Verification items for the finished model (mm, model axes). A direction names the side the tool comes from. Give positions to 0.01 mm unless a question says otherwise; leave off trailing zeros. Loops run counter-clockwise (first coordinate to the right, second up) from the corner with the lowest first, then second, coordinate; pieces in that order, holes last. Notation, with made-up numbers: (62.5, 20.5) - (79.5, 20.5) arc R16 ccw to (79.5, 45.5) - close; hole circle Ø3 at (-27.5, 72). An arc over 180 degrees is marked (long way). Use one line per item in the form item = value.
```python
from build123d import *

# Parameters (mm, degrees)
SKETCH1_R                = 300
BOSS_EXTRUDE1_DEPTH      = 161
SKETCH2_R                = 192.75
SKETCH2_R_2              = 100
SKETCH2_W                = 642.75
SKETCH2_H                = 214
BOSS_EXTRUDE2_DEPTH      = 50
SKETCH3_R                = 75
CUT_EXTRUDE1_DEPTH       = 40
SKETCH4_R                = 100
CUT_EXTRUDE2_DEPTH       = 40
BOSS_EXTRUDE3_REACH      = 982.366
BOSS_EXTRUDE3_END_RADIUS = 192.75
SKETCH5_W                = 100
SKETCH5_H                = 83.75


with BuildPart() as part:
    # Sketch1 → Boss-Extrude1 (new body)
    with BuildSketch(Plane(origin=(0, 0, 0), x_dir=(1, 0, 0), z_dir=(0, 1, 0))):
        with Locations(Location((0, 0, 0), (0, 0, 270))):
            Circle(SKETCH1_R)
    extrude(amount=BOSS_EXTRUDE1_DEPTH)

    # Sketch2 → Boss-Extrude2 (add, symmetric)
    # profile 1 of 2: a face of its own
    with BuildSketch(Plane.XY):
        with Locations((330, 484)):
            Circle(SKETCH2_R)
        with Locations((330, 484)):
            Circle(SKETCH2_R_2, mode=Mode.SUBTRACT)
    # profile 2 of 2: a face of its own
    with BuildSketch(Plane.XY):
        with Locations((-201.375, 268)):
            Rectangle(SKETCH2_W, SKETCH2_H)
    extrude(amount=BOSS_EXTRUDE2_DEPTH, both=True)


with BuildPart() as boss_extrude2_piece_1:
    # of the separate pieces the step leaves, piece 1, a body of its own (boss_extrude2_pieces)
    add(part.part.solids().sort_by_distance((0, 0, 300))[0])

    # Sketch3 → Cut-Extrude1 (cut)
    with BuildSketch(Plane.XZ):
        with Locations(Location((0, 0, 0), (0, 0, 270))):
            Circle(SKETCH3_R)
    extrude(amount=-CUT_EXTRUDE1_DEPTH, mode=Mode.SUBTRACT)

    # Sketch4 → Cut-Extrude2 (cut)
    with BuildSketch(Plane.XZ.offset(-40)):
        with Locations(Location((0, 0, 0), (0, 0, 270))):
            Circle(SKETCH4_R)
    extrude(amount=-CUT_EXTRUDE2_DEPTH, mode=Mode.SUBTRACT)



with BuildPart() as boss_extrude2_piece_2:
    # of the separate pieces the step leaves, piece 2, a body of its own (boss_extrude2_pieces)
    add(part.part.solids().sort_by_distance((522.75, 484, -50))[0])


with BuildPart() as boss_extrude2_piece_1_1:
    add(boss_extrude2_piece_1.part)

    add(boss_extrude2_piece_2.part)  # Boss-Extrude3 merges Boss-Extrude2 piece 2
    # Boss-Extrude3: up to this cylinder (the profile starts outside it)
    boss_extrude3_end = Plane(origin=(330, 484, 0), z_dir=(0, 0, -1)) * Cylinder(BOSS_EXTRUDE3_END_RADIUS, 2351.232, mode=Mode.PRIVATE)
    # Sketch5 → Boss-Extrude3 (add, up to the surface)
    with BuildSketch(Plane(origin=(120, 0, 0), x_dir=(0, 0, -1), z_dir=(1, 0, 0)), mode=Mode.PRIVATE) as boss_extrude3_sk1:
        with Locations((0, 333.125)):
            Rectangle(SKETCH5_W, SKETCH5_H)
    boss_extrude3_tool1 = extrude(boss_extrude3_sk1.sketch, amount=BOSS_EXTRUDE3_REACH, mode=Mode.PRIVATE) - boss_extrude3_end
    add(boss_extrude3_tool1.solids().sort_by_distance((120, 333.125, 0))[0])


solid = boss_extrude2_piece_1_1.part
```
1. Section check A-A, the plane y = 484. Record the cut outline in (x, z).
Result set:
outline = (137.25, -50) - (230, -50) - (230, 50) - (137.25, 50) - close; (430, -50) - (522.75, -50) - (522.75, 50) - (430, 50) - close
2. Depth check by flat-ended pin: pin 1 Ø3 at (y, z) = (407.5, -7.5) entering from -X; pin 2 Ø4 at (x, z) = (-262, 78) entering from -Y; pin 3 Ø2 at (x, z) = (-403.5, 50.5) entering from -Y. Enter the tip coordinate at first touch or a pass-through.
Result set:
pin_1 = 152.44
pin_2 = 0
pin_3 = 161
3. Tool access check on faces 4 (the flat face through (-522.75, 267, 1)), 5 (the flat face through (-7, 358, -50)), 6 (the flat face through (1, 80, 1)), 7 (the flat face through (120, 225, 1)), 8 (the flat face through (-7, 358, 50)). Record the directions out of +Z, -Z, +X, -X, +Y, -Y that give a thin tool (end or side, any length) a straight path to the whole face; none if there is none.
Result set:
face_4 = +Z, -Z, -X, +Y, -Y
face_5 = -Z, +X, -X, +Y
face_6 = none
face_7 = +Z, -Z, +X
face_8 = +Z, +X, -X, +Y
4. Section check B-B, the plane z = 0. Record the cut outline in (x, y).
Result set:
outline = (-522.75, 161) - (-300, 161) - (-300, 0) - (-75, 0) - (-75, 40) - (-100, 40) - (-100, 80) - (100, 80) - (100, 40) - (75, 40) - (75, 0) - (300, 0) - (300, 161) - (120, 161) - (120, 291.25) - (330, 291.25) arc R192.75 ccw (long way) to (171.03, 375) - (-522.75, 375) - close; hole circle Ø200 at (330, 484)
5. Scan lines: probe 1 along X at (y, z) = (20, 0); probe 2 along Y at (x, z) = (330, -5); probe 3 along Y at (x, z) = (-450, -10). Record each from-to range of solid material in increasing order.
Result set:
probe_1 = -300 to -75, 75 to 300
probe_2 = 291.25 to 384, 584 to 676.75
probe_3 = 161 to 375
6. Section check C-C, the plane x = 0. Record the cut outline in (y, z).
Result set:
outline = (0, -300) - (161, -300) - (161, -50) - (375, -50) - (375, 50) - (161, 50) - (161, 300) - (0, 300) - (0, 75) - (40, 75) - (40, 100) - (80, 100) - (80, -100) - (40, -100) - (40, -75) - (0, -75) - close
7. Section check D-D, the plane y = 186. Record the cut outline in (x, z), then the cut area to 3 significant figures.
Result set:
outline = (-522.75, -50) - (120, -50) - (120, 50) - (-522.75, 50) - close
area = 64,300 mm²
8. Draft check along Y on faces 1 (the flat face through (-62, 0, 62)), 2 (the cylindrical face through (-45.636, 19.72, 59.517)), 3 (the cylindrical face through (256.296, 551.585, -0.7)). Enter one of: released by +Y, released by -Y, zero draft, split by the parting line, or undercut.
Result set:
face_1 = released by -Y
face_2 = zero draft
face_3 = undercut
